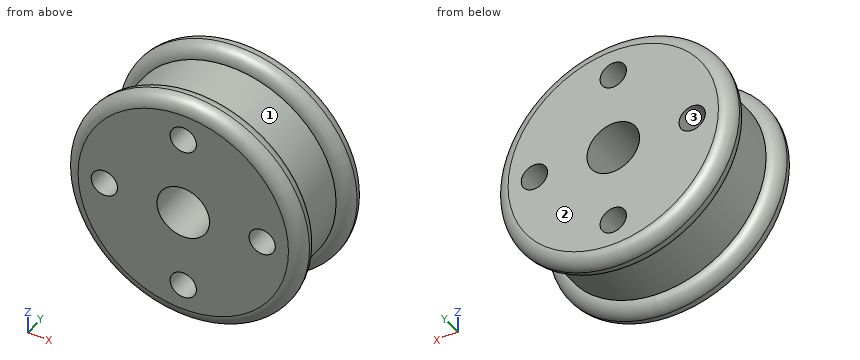
from build123d import *

# Parameters (mm, degrees)
F0_R     = 25.4
F1_DEPTH = 12.7
F2_R     = 28.575
F3_DEPTH = 6.35
F4_R     = 28.575
F5_DEPTH = 6.35
F6_R     = 6.35
F7_DEPTH = 25.401
F9_D     = 6.35
F10_R    = 3.17499


# Not quite as in the source:
# - a fillet or chamfer is up to 0.001 mm smaller than in the source, because OpenCascade refuses the exact size


with BuildPart() as f1:
    # F0 (on Front) → F1 (new body)
    with BuildSketch(Plane.XZ):
        Circle(F0_R)
    extrude(amount=F1_DEPTH)

    # F2 (on face) → F3 (join)
    with BuildSketch(Plane.XZ.offset(12.7)):
        Circle(F2_R)
    extrude(amount=F3_DEPTH)

    # F4 (on face) → F5 (join)
    with BuildSketch(Plane(origin=(0, 0, 0), x_dir=(-1, 0, 0), z_dir=(0, 1, 0))):
        Circle(F4_R)
    extrude(amount=F5_DEPTH)

    # F6 (on face) → F7 (cut, through all)
    with BuildSketch(Plane(origin=(0, 6.35, 0), x_dir=(-1, 0, 0), z_dir=(0, 1, 0))):
        Circle(F6_R)
    extrude(amount=-F7_DEPTH, mode=Mode.SUBTRACT)

    # F9 (through all)
    with Locations(Plane(origin=(0, 6.35, 0), x_dir=(-1, 0, 0), z_dir=(0, 1, 0))):
        with Locations((0, 19.05), (19.05, 0), (0, -19.05), (-19.05, 0)):
            Hole(F9_D / 2)

    # F10 (radius 3.175 in the source; OpenCascade refuses exactly that, so slightly less here)
    f10_edges = [f1.edges().sort_by_distance(p)[0] for p in [
        (28.575, 6.35, 0),
        (28.575, 0, 0),
        (-28.575, -12.7, 0),
        (-28.575, -19.05, 0),
    ]]
    fillet(f10_edges, radius=F10_R)


solid = f1.part
Source: CAD feature listing. Evaluate the final solid. Frame: model axes, mm. Face numbers are marked on the shaded views. Give positions to 0.01 mm unless a question says otherwise; leave off trailing zeros. Loops run counter-clockwise (first coordinate to the right, second up) from the corner with the lowest first, then second, coordinate; pieces in that order, holes last. Notation, with made-up numbers: (72, -10) -> (131, -10) arc R31 cw to (131, 23) -> close; hole circle Ø10 at (32, 55.5). An arc over 180 degrees is marked (long way). Use a Markdown table: item, result. Add a question column.
1) Section query A-A, the plane x = 0. Count the separate pieces of the cut face and the enclosed holes in it, then the cut area to 4 significant figures.
2) Section query D-D, the plane y = -14. Return the cut outline in (x, z) (3 decimals).
3) Line query: line 1 along Z through (x, y) = (-1.5, -9.5); line 2 along X through (y, z) = (-17.25, -2); line 3 along X through (y, z) = (-13.25, -0.5). Output: solid intervals per line, ascending. Write a range as [from, to].
4) Section query C-C, the plane y = -7. Return the cut outline in (x, z) (3 decimals).
5) First-contact query: pin 1 (12 mm diameter, centred on y = -9, z = -7, fed in from +X); pin 2 (5 mm diameter, centred on y = -11.5, z = -13.5, fed in from +X); pin 3 (5 mm diameter, centred on x = -6.5, y = -12.5, fed in from -Z). Flat tips, straight axial feed; report the tip coordinate or a pass-through.
6) Pull-direction query (X, two-part tool) for the marked faces 1, 2 and 3; classes: +X half, -X half, draft (parallel to the pull), parting line (faces both ways), or undercut.
Numbers:
| question | item | result |
|---|---|---|
| 1 | separate pieces | 4 |
| 1 | enclosed holes | 0 |
| 1 | area | 708.5 mm2 |
| 2 | outline | circle Ø55.924 at (0, 0); hole circle Ø6.35 at (-19.05, 0); hole circle Ø12.7 at (0, 0); hole circle Ø6.35 at (0, -19.05); hole circle Ø6.35 at (0, 19.05); hole circle Ø6.35 at (19.05, 0) |
| 3 | line 1 | z = [-25.36, -21.85], [-16.25, -6.17], [6.17, 16.25], [21.85, 25.36] |
| 3 | line 2 | x = [-28.19, -21.52], [-16.58, -6.03], [6.03, 16.58], [21.52, 28.19] |
| 3 | line 3 | x = [-27.18, -22.19], [-15.91, -6.33], [6.33, 15.91], [22.19, 27.18] |
| 4 | outline | circle Ø50.8 at (0, 0); hole circle Ø6.35 at (-19.05, 0); hole circle Ø12.7 at (0, 0); hole circle Ø6.35 at (0, -19.05); hole circle Ø6.35 at (0, 19.05); hole circle Ø6.35 at (19.05, 0) |
| 5 | pin 1 | stops at x = 27.89 |
| 5 | pin 2 | stops at x = 24.83 |
| 5 | pin 3 | stops at z = -27.85 |
| 6 | face 1 | parting line |
| 6 | face 2 | draft |
| 6 | face 3 | undercut |
